from build123d import *

# Parameters (mm, degrees)
SKETCH1_W           = 15
SKETCH1_H           = 20
BOSS_EXTRUDE1_DEPTH = 3
SKETCH2_R           = 0.7
BOSS_EXTRUDE2_DEPTH = 14
SKETCH2_2_R         = 0.7
CUT_EXTRUDE1_DEPTH  = 6
CUT_EXTRUDE2_START  = -2
CUT_EXTRUDE2_DEPTH  = 2
CUT_EXTRUDE3_DEPTH  = 2


with BuildPart() as part:
    # Sketch1 → Boss-Extrude1 (new body)
    with BuildSketch(Plane.XY):
        Rectangle(SKETCH1_W, SKETCH1_H)
    extrude(amount=BOSS_EXTRUDE1_DEPTH)

    # Sketch2 → Boss-Extrude2 (add)
    with BuildSketch(Plane(origin=(0, 10, 0), x_dir=(1, 0, 0), z_dir=(0, 1, 0))):
        with BuildLine():
            Line((-5, -3), (-5, -13.5))
            ThreePointArc((-5, -13.5), (0, -18.5), (5, -13.5))
            Line((5, -13.5), (5, -3))
            Line((5, -3), (-5, -3))
        make_face()
        with Locations(Location((0, -13.5, 0), (0, 0, 270))):
            Circle(SKETCH2_R, mode=Mode.SUBTRACT)
    extrude(amount=-BOSS_EXTRUDE2_DEPTH)

    # Sketch2_2 → Cut-Extrude1 (cut)
    with BuildSketch(Plane(origin=(0, 10, 0), x_dir=(1, 0, 0), z_dir=(0, 1, 0))):
        with BuildLine():
            Line((-5, -3), (-5, -13.5))
            ThreePointArc((-5, -13.5), (0, -18.5), (5, -13.5))
            Line((5, -13.5), (5, -3))
            Line((5, -3), (-5, -3))
        make_face()
        with Locations(Location((0, -13.5, 0), (0, 0, 270))):
            Circle(SKETCH2_2_R, mode=Mode.SUBTRACT)
    extrude(amount=-CUT_EXTRUDE1_DEPTH, mode=Mode.SUBTRACT)

    # Sketch3 → Cut-Extrude2 (cut)
    with BuildSketch(Plane.XZ.offset(4).offset(CUT_EXTRUDE2_START)):
        with BuildLine():
            Line((5, 13.5), (5, 3))
            Line((5, 3), (-5, 3))
            Line((-5, 3), (-5, 13.5))
            ThreePointArc((-5, 13.5), (0, 18.5), (5, 13.5))
        make_face()
    extrude(amount=CUT_EXTRUDE2_DEPTH, mode=Mode.SUBTRACT)

    # Sketch4 → Cut-Extrude3 (cut)
    with BuildSketch(Plane(origin=(0, 4, 0), x_dir=(1, 0, 0), z_dir=(0, 1, 0))):
        with BuildLine():
            Line((-5, -13.5), (-5, -3))
            Line((-5, -3), (5, -3))
            Line((5, -3), (5, -13.5))
            ThreePointArc((5, -13.5), (0, -18.5), (-5, -13.5))
        make_face()
    extrude(amount=-CUT_EXTRUDE3_DEPTH, mode=Mode.SUBTRACT)


solid = part.part
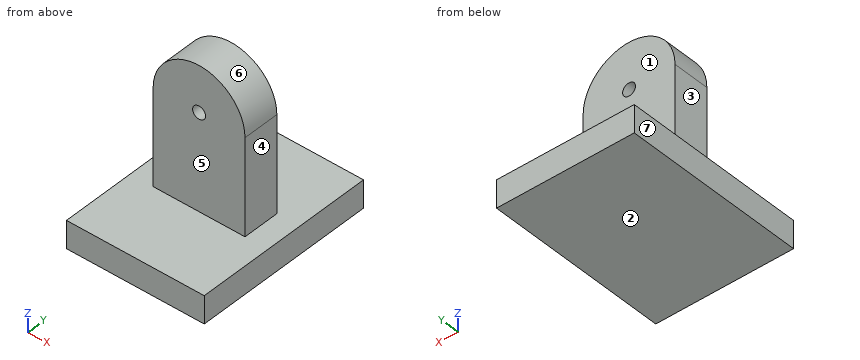
Can you work these out from the model? Positions are in its coordinate system, mm. Face numbers are marked on the shaded views. A direction names the side the tool comes from. Coordinates: 2 decimals unless noted, no trailing zeros. Loops run counter-clockwise (first coordinate to the right, second up) from the corner with the lowest first, then second, coordinate; pieces in that order, holes last. Notation, with made-up numbers: M 35,60.5 L 43,60.5 A28 ccw 43,97.5 Z; hole C 29.5,39 d3. An arc over 180 degrees is marked long. Answer as CSV lines item,"result". Start each with the question number.
1. For pin 1 Ø8 at (x, z) = (-2, 12.5) entering from -Y; pin 2 Ø2 at (y, z) = (-1, 7.5) entering from +X; pin 3 Ø2 at (x, z) = (5.5, 9) entering from +Y; pin 4 Ø1.1 at (x, z) = (0, 13.5) entering from +Y, each with a flat end and sliding along its axis, tell me the tip position at first contact or that it passes through.
2. Suppose I cut it at C-C, the plane x = 3. List the corners of the cut face in (y, z) for me, plus the area to 3 significant figures.
3. Thinking about a two-plate mould opening in X: for the marked faces 4, 5, 6 and 7, which applies, +X half, -X half, draft (parallel to the pull), parting line (faces both ways), or undercut?
4. If I drill on probe 1 along X at (y, z) = (-0.25, 13.5); probe 2 along Y at (x, z) = (4.25, 6.75); probe 3 along Z at (x, y) = (-3.75, -5.25), over which ranges is the centre line in solid material (lowest first)? Write a range as [from, to].
5. Suppose I cut it at B-B, the plane y = 1.25. List the corners of the cut face in (x, z) for me.
6. Suppose I cut it at A-A, the plane x = 0. List the corners of the cut face in (y, z) for me.
7. Suppose I cut it at D-D, the plane z = 10. List the corners of the cut face in (x, y) for me.
8. For the marked faces 1, 2 and 3, which set-ups out of +Z, -Z, +X, -X, +Y, -Y let a thin tool reach every point of the face, with its end or its side?
Output:
1,pin 1,"stops at y = -2"
1,pin 2,"stops at x = 5"
1,pin 3,"stops at y = 2"
1,pin 4,"passes through"
2,outline,"M -10,0 L 10,0 L 10,3 L 2,3 L 2,17.5 L -2,17.5 L -2,3 L -10,3 Z"
2,area,"118 mm^2"
3,face 4,"+X half"
3,face 5,"draft"
3,face 6,"parting line"
3,face 7,"-X half"
4,probe 1,"x = [-5, -0.7], [0.7, 5]"
4,probe 2,"y = [-2, 2]"
4,probe 3,"z = [0, 3]"
5,outline,"M -7.5,0 L 7.5,0 L 7.5,3 L 5,3 L 5,13.5 A5 ccw -5,13.5 L -5,3 L -7.5,3 Z; hole C 0,13.5 d1.4"
6,outline,"M -10,0 L 10,0 L 10,3 L 2,3 L 2,12.8 L -2,12.8 L -2,3 L -10,3 Z; M -2,14.2 L 2,14.2 L 2,18.5 L -2,18.5 Z"
7,outline,"M -5,-2 L 5,-2 L 5,2 L -5,2 Z"
8,face 1,"+Z, +X, -X, +Y"
8,face 2,"-Z, +X, -X, +Y, -Y"
8,face 3,"+Z, -X, +Y, -Y"
